from build123d import *

# Parameters (mm, degrees)
SKETCH_1_W          = 62.4134
SKETCH_1_H          = 16.3
EXTRUDE_1_DEPTH     = 4
SKETCH_3_W          = 70.55
SKETCH_3_H          = 16.3
SKETCH_3_R          = 1.55
EXTRUDE_3_DEPTH     = 4
CUT_EXTRUDE_1_REACH = 77.702
SKETCH_4_R          = 0.6


with BuildPart() as part:
    # 草图1 → 凸台-拉伸1 (new body)
    with BuildSketch(Plane.XY):
        with Locations((-3.9433, 0)):
            Rectangle(SKETCH_1_W, SKETCH_1_H)
    extrude(amount=EXTRUDE_1_DEPTH)

    # 草图3 → 凸台-拉伸3 (add)
    with BuildSketch(Plane.ZY.offset(35.15)):
        with Locations((-31.275, 0)):
            Rectangle(SKETCH_3_W, SKETCH_3_H)
        with Locations((-56.55, 0.5)):
            Circle(SKETCH_3_R, mode=Mode.SUBTRACT)
        with Locations((-18.75, 0.5)):
            Circle(SKETCH_3_R, mode=Mode.SUBTRACT)
    extrude(amount=-EXTRUDE_3_DEPTH)

    # 草图4 → 切除-拉伸1 (cut, up to next)
    with BuildSketch(Plane(origin=(0, 0, 0), x_dir=(-1, 0, 0), z_dir=(0, 0, -1)), mode=Mode.PRIVATE) as cut_extrude_1_sk1:
        with Locations((-22.75, -4.52)):
            Circle(SKETCH_4_R)
    cut_extrude_1_tool1 = extrude(cut_extrude_1_sk1.sketch, amount=-CUT_EXTRUDE_1_REACH, mode=Mode.PRIVATE) & part.part
    # 草图4 → 切除-拉伸1 (cut, up to next)
    with BuildSketch(Plane(origin=(0, 0, 0), x_dir=(-1, 0, 0), z_dir=(0, 0, -1)), mode=Mode.PRIVATE) as cut_extrude_1_sk2:
        with Locations((13.65, -4.52)):
            Circle(SKETCH_4_R)
    cut_extrude_1_tool2 = extrude(cut_extrude_1_sk2.sketch, amount=-CUT_EXTRUDE_1_REACH, mode=Mode.PRIVATE) & part.part
    add(cut_extrude_1_tool1.solids().sort_by_distance((22.75, -4.52, 0))[0], mode=Mode.SUBTRACT)
    add(cut_extrude_1_tool2.solids().sort_by_distance((-13.65, -4.52, 0))[0], mode=Mode.SUBTRACT)


solid = part.part
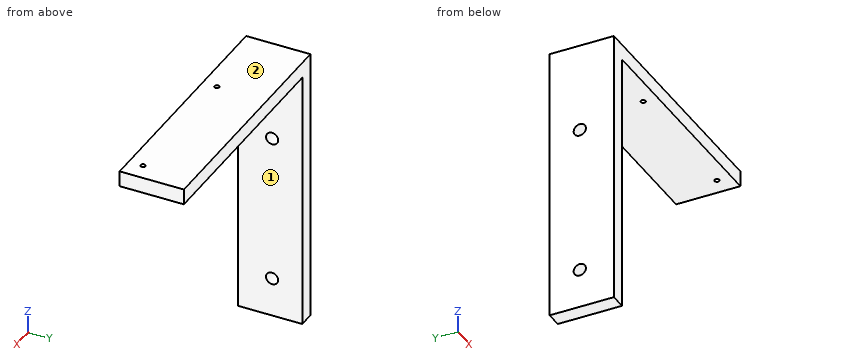
For this review, take the finished solid that the model builds, in its own axes (mm). Face numbers are marked on the shaded views. A direction names the side the tool comes from. Give positions to 0.01 mm unless a question says otherwise; leave off trailing zeros. Loops run counter-clockwise (first coordinate to the right, second up) from the corner with the lowest first, then second, coordinate; pieces in that order, holes last.
Item 1: Tool access review of the marked faces 1 and 2: name each direction out of +Z, -Z, +X, -X, +Y, -Y from which nothing blocks a thin tool from reaching the whole face with its end or side.
Item 2: For line 1 along Y through (x, z) = (-13.65, 3); line 2 along Y through (x, z) = (-33.35, -56.55); line 3 along X through (y, z) = (0.25, -20.5), list the stretches that pass through material, from the lowest coordinate up.
Item 3: Insertion check: pin 1 (5 mm diameter, centred on y = -4.5, z = -32, fed in from +X); pin 2 (4 mm diameter, centred on x = -6, y = -0.5, fed in from -Z); pin 3 (5 mm diameter, centred on y = 0.5, z = -56.55, fed in from -X). Each pin has a flat end and moves straight along its axis. Give the tip position at first contact, or say it passes through.
Item 4: Take a section at C-C, the plane x = -16.5. State the section outline as (y, z) points, and give its area (3 significant figures).
Item 5: Take a section at D-D, the plane y = 4.5. State the section outline as (x, z) points, and give its area (3 significant figures).
Item 6: Take a section at A-A, the plane z = -18.75. State the section outline as (x, y) points, and give its area (3 significant figures).
Item 7: Take a section at B-B, the plane y = 0.5. State the section outline as (x, z) points, and give its area (3 significant figures).
Calculated:
1. face 1: -Z, +X, +Y, -Y
1. face 2: +Z, +X, -X, +Y, -Y
2. line 1: y = -8.15 to -5.12, -3.92 to 8.15
2. line 2: y = -8.15 to -1.05, 2.05 to 8.15
2. line 3: x = -35.15 to -31.15
3. pin 1: stops at x = -31.15
3. pin 2: stops at z = 0
3. pin 3: stops at x = -35.15
4. outline: (-8.15, 0) - (8.15, 0) - (8.15, 4) - (-8.15, 4) - close
4. area: 65.2 mm2
5. outline: (-35.15, -66.55) - (-31.15, -66.55) - (-31.15, 0) - (27.26, 0) - (27.26, 4) - (-35.15, 4) - close
5. area: 516 mm2
6. outline: (-35.15, -8.15) - (-31.15, -8.15) - (-31.15, -1.05) - (-35.15, -1.05) - close; (-35.15, 2.05) - (-31.15, 2.05) - (-31.15, 8.15) - (-35.15, 8.15) - close
6. area: 52.8 mm2
7. outline: (-35.15, -66.55) - (-31.15, -66.55) - (-31.15, -58.1) - (-35.15, -58.1) - close; (-35.15, -55) - (-31.15, -55) - (-31.15, -20.3) - (-35.15, -20.3) - close; (-35.15, -17.2) - (-31.15, -17.2) - (-31.15, 0) - (27.26, 0) - (27.26, 4) - (-35.15, 4) - close
7. area: 491 mm2
